For this review, take the finished solid that the model builds, in its own axes (mm). Face numbers are marked on the shaded views. Coordinates: 2 decimals unless noted, no trailing zeros. Order: outer loops, then holes, each group sorted by start corner. A loop starts at its lowest first (then second) coordinate and runs counter-clockwise, first axis right, second up. Notation, with made-up numbers: (85.25, 29.25) -> (100.25, 29.25) arc R19 cw to (100.25, 42.25) -> close; hole circle Ø5 at (-4.5, 6.5). An arc over 180 degrees is marked (long way). Write item = value, one per line. Start each with the question number.
1) Wall thickness on probe 1 along Z at (x, y) = (17.75, 0); probe 2 along X at (y, z) = (2, -1.25); probe 3 along X at (y, z) = (-1.5, 1.5): over which ranges is each line inside the solid? List them lowest first. Write a range as [from, to].
2) Consider section A-A on x = 13.5. Give the boundary of the cut face in (y, z).
3) Insertion check: pin 1 Ø1 at (x, z) = (11.5, -1.5) entering from +Y; pin 2 Ø1.3 at (x, z) = (-1, 0) entering from -Y; pin 3 Ø0.6 at (x, z) = (-1.5, 0) entering from +Y. Each pin has a flat end and moves straight along its axis. Give the tip position at first contact, or say it passes through.
4) Draft analysis for pull direction Z (two halves, no side actions). For the marked faces 1, 2 and 3, state which applies: +Z half, -Z half, draft (parallel to the pull), parting line (faces both ways), or undercut.
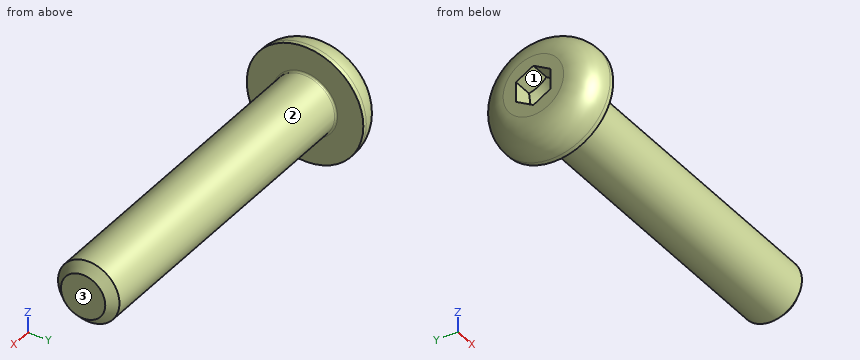
Autodesk Inventor part; units mm, degrees
ref_plane "Work Plane1" through (29, 0, 0) normal (0, -1, 0) x (1, 0, 0)
ref_plane "YZ Plane" through (0, 0, 0) normal (1, 0, 0) x (0, 1, 0)
ref_plane "XZ Plane" through (0, 0, 0) normal (0, 1, 0) x (-1, 0, 0)
sketch "Sketch1" plane through (0, 0, 0) normal (0, 0, 1) x (1, 0, 0)
  line L0 (-0.0762, 0) -> (19.05, 0)
  line L1 (19.05, 0) -> (19.05, 1.7526)
  line L2 (19.05, 1.7526) -> (1.5902, 1.7526)
  line L3 (1.5902, 1.7526) -> (0.0001, 1.7526)
  line L4 (0.0001, 1.7526) -> (0, 1.7526)
  line L5 (0, 1.7526) -> (0, 3.3274)
  line L6 (0, 3.3274) -> (-1.8542, 3.3274)
  line L7 (-1.8542, 3.3274) -> (-1.8542, 1.1438)
  line L8 (-1.8542, 1.1438) -> (-0.7366, 1.1438)
  line L9 (-0.7366, 1.1438) -> (-0.0762, 0)
  line L10 (-6.035, 0) -> (23.2308, 0)
  line L11 (0, -0.6655) -> (0, 3.9929)
  line L12 (1.5902, 1.7526) -> (0, 1.7526) construction
  dimension "d1" = 17.4598
  dimension "d2" = 1.5901
  dimension "d3" = 1.8542
  dimension "d4" = 1.1176
  dimension "d5" = 60
  dimension "d6" = 3.5052
  dimension "d7" = 3.5052
  dimension "d8" = 2.2877
  dimension "d9" = 6.6548
  dimension "d26" = 19.05
revolve "Body" add sketch "Sketch1" angle 360 about axis through (-0.0762, 0, 0) along (1, 0, 0)
sketch "Sketch2" plane through (-1.8542, 0, 0) normal (-1, 0, 0) x (0, 0, 1)
  circle A0 centre (0, 0) radius 1.1438
  line L0 (0, -4.6584) -> (0, 4.6584)
  line L1 (-4.6584, 0) -> (4.6584, 0)
  line L2 (1.1438, 0) -> (0.5719, -0.9906)
  line L3 (0.5719, -0.9906) -> (-0.5719, -0.9906)
  line L4 (-0.5719, -0.9906) -> (-1.1438, 0)
  line L5 (-1.1438, 0) -> (-0.5719, 0.9906)
  line L6 (-0.5719, 0.9906) -> (0.5719, 0.9906)
  line L7 (0.5719, 0.9906) -> (1.1438, 0)
extrude "Slot" add sketch "Sketch2" against normal up to next contours L7 A0 | A0 L2 | L6 L0 A0 | A0 L0 L3 | L0 L6 A0 | A0 L3 L0 | L4 A0 | A0 L5
fillet "Fillet1" radius 1.6002 1 edges at (-1.8542, -3.3274, 0)
thread "Thread"
chamfer "Chamfer1" distance 0.4869 distance2 0.4869 1 edges at (19.05, -1.7526, 0) measured on face at (19.05, 0.4373, -0.3874)
ref_plane "Work Plane1" through (29, 0, 0) normal (0, -1, 0) x (1, 0, 0)
fillet "Fillet2" radius 0.1 1 edges at (0.0001, -1.7526, 0)
equation "\"d1\" = GEL"
equation "\"d3\" = KOH"
equation "\"d4\" = INTI"
equation "\"d6\" = GD"
equation "\"d7\" = BDM"
equation "\"d8\" = 1.1547 * SW"
equation "\"d9\" = KOD"
equation "\"d26\" = NLG"
equation "\"d30\" = R"
equation "\"d17\" = RR"
equation "\"d13\" = GEL"
equation "\"d15\" = -0.5 * SPD + 0.5 * GD"
equation "\"d16\" = GUL"
equation "\"GD\" = NND"
equation "\"NLG\" = 19.05"
equation "\"GEL\" = 17.45976"
equation "\"KOD\" = 6.6548"
equation "\"KOH\" = 1.8542"
equation "\"INTI\" = 1.1176"
equation "\"GAL\" = 1.59004"
equation "\"GUL\" = 0.48692"
equation "\"BDM\" = NND"
equation "\"SW\" = 1.9812"
equation "\"RR\" = 1.6002"
equation "\"SPD\" = 2.53136"
equation "\"R\" = 0.1"
equation "\"TOA\" = 30deg"
equation "\"GD1\" = SPD"
equation "\"THREADDIA\" = 3.5052"
equation "\"KOH1\" = 0.381"
equation "\"NND\" = 3.5052"
equation "\"E0\" = 2.28829"
properties part number "ANSI B18.3 - 6 - 32 x 3/4" material "Steel, Mild"
Answer sheet:
q1.probe_1 = [-1.75, 1.75]
q1.probe_2 = [-1.72, 0]
q1.probe_3 = [-1.8, 0]
q2.outline = circle Ø3.51 at (0, 0)
q3.pin_1 = 1.44
q3.pin_2 = -3.32
q3.pin_3 = 3.02
q4.face_1 = undercut
q4.face_2 = parting line
q4.face_3 = draft
